```python
from build123d import *

# Parameters (mm, degrees)
F0_W     = 4.7625
F0_H     = 33.3375
F1_DEPTH = 19.05
F2_SIZE  = 5.08
F3_DEPTH = 38.1
F4_R     = 3.175
F4_R_2   = 1.5875
F5_DEPTH = 0.79375
F6_DEPTH = 4.7625


with BuildPart() as f1:
    # F0 (on Top) → F1 (new body)
    with BuildSketch(Plane.XY):
        Polygon((-25.4, 30.1625), (-25.4, 25.4), (-20.6375, 25.4), (25.4, 25.4), (25.4, 30.1625), align=None)
        Polygon((-20.6375, 25.4), (-25.4, 25.4), (-25.4, -58.7375), (-20.6375, -58.7375), (-20.6375, -53.975), align=None)
        Polygon((26.9875, -53.975), (-20.6375, -53.975), (-20.6375, -58.7375), (31.75, -58.7375), (31.75, -53.975), align=None)
        with Locations((29.36875, -37.30625)):
            Rectangle(F0_W, F0_H)
    extrude(amount=F1_DEPTH)

    # F2
    f2_edges = [f1.edges().sort_by_distance(p)[0] for p in [
        (-20.6375, -53.975, 9.525),
        (-20.6375, 25.4, 9.525),
        (26.9875, -53.975, 9.525),
    ]]
    chamfer(f2_edges, length=F2_SIZE)

    # F0 (on Top) → F3 (join)
    with BuildSketch(Plane.XY):
        Polygon((-25.4, 30.1625), (-25.4, 25.4), (-20.6375, 25.4), (25.4, 25.4), (25.4, 30.1625), align=None)
    extrude(amount=F3_DEPTH)

    # F4 (on face) → F5 (cut)
    with BuildSketch(Plane.XZ.offset(-25.4)):
        with Locations((-12.7, 28.575)):
            Circle(F4_R)
        with Locations((-12.7, 28.575)):
            Circle(F4_R_2, mode=Mode.SUBTRACT)
        with Locations((12.7, 28.575)):
            Circle(F4_R)
        with Locations((12.7, 28.575)):
            Circle(F4_R_2, mode=Mode.SUBTRACT)
    extrude(amount=-F5_DEPTH, mode=Mode.SUBTRACT)

    # F6 (cut, through all): faces of the model
    f6_faces = [f1.faces().sort_by_distance(p)[0] for p in [
        (-12.7, 25.4, 28.575),
        (12.7, 25.4, 28.575),
    ]]
    extrude(f6_faces, amount=-F6_DEPTH, mode=Mode.SUBTRACT)


solid = f1.part
```
Input: part model. Units: mm. Frame: model coordinates. A direction names the side the tool comes from. Give positions to 0.01 mm unless a question says otherwise; leave off trailing zeros. Order: outer loops, then holes, each group sorted by start corner. A loop starts at its lowest first (then second) coordinate and runs counter-clockwise, first axis right, second up. Notation, with made-up numbers: M 57.5,71 L 63.5,71 A5 cw 63.5,75 Z; hole C 33,28 d8. An arc over 180 degrees is marked long. Return JSON: item names as keys, results as strings.
1) Section query B-B on x = 12.7. Count the separate pieces of the cut face and the enclosed holes in it, and give its area (3 significant figures).
Taken from the geometry:
{"separate pieces": "3", "enclosed holes": "0", "area": "255 mm2"}
2) Contact query for flat-ended pins moving along their axis: pin 1 (2 mm diameter, centred on x = 21.5, z = 22, fed in from -Y); pin 2 (5 mm diameter, centred on y = -47, z = 19.5, fed in from -X); pin 3 (1.9 mm diameter, centred on x = 13.5, z = 29, fed in from -Y); pin 4 (2.5 mm diameter, centred on y = 28, z = 25.5, fed in from +X). Output: stop coordinate, or through.
Taken from the geometry:
{"pin 1": "stops at y = 25.4", "pin 2": "stops at x = -25.4", "pin 3": "stops at y = 26.19", "pin 4": "stops at x = 25.4"}
3) Line query: L1, parallel to Y at x = 1.5, z = 7.5 (1 decimal); L2, parallel to Z at x = -12.7, y = 29.25; L3, parallel to Y at x = -9, z = 26.5. Output: solid intervals per line, ascending. Write a range as [from, to].
Taken from the geometry:
{"L1": "y = [-58.7, -54], [25.4, 30.2]", "L2": "z = [0, 26.99], [30.16, 38.1]", "L3": "y = [25.4, 30.16]"}
4) Section query A-A on y = -42. Output: boundary loops of the cut face in (x, z).
Taken from the geometry:
{"outline": "M -25.4,0 L -20.64,0 L -20.64,19.05 L -25.4,19.05 Z; M 26.99,0 L 31.75,0 L 31.75,19.05 L 26.99,19.05 Z"}
5) Access query for faces 4 (the face through (-22, -14, 0)), 5 (the face through (11, 26.194, 28)), 6 (the face through (29, -20.638, 9)), 7 (the face through (-18.13, -51.4, 9.39)), 8 (the face through (-22, -29, 19.05)). Directions: +Z, -Z, +X, -X, +Y, -Y. A direction counts if a zero-diameter tool reaches every point of the face in a straight line with its end or side. Return the directions, or none.
Taken from the geometry:
{"face 4": "-Z, +X, -X, +Y, -Y", "face 5": "-Y", "face 6": "+Z, -Z, +X, +Y", "face 7": "+Z, -Z", "face 8": "+Z, +X, -X, -Y"}
6) Mould query, pull axis X, two halves, no side actions, for faces 1 (the face through (3, -53.975, 9)), 2 (the face through (5, 25.4, 19)), 3 (the face through (-18.06, 22.9, 9.39)). Classes: released by +X, released by -X, zero draft, split by the parting line, or undercut.
Taken from the geometry:
{"face 1": "undercut", "face 2": "zero draft", "face 3": "released by +X"}
